Work out the finished part from the listing and answer in its coordinate system (mm). Face numbers are marked on the shaded views. A direction names the side the tool comes from. Coordinates: 2 decimals unless noted, no trailing zeros. Order: outer loops, then holes, each group sorted by start corner. A loop starts at its lowest first (then second) coordinate and runs counter-clockwise, first axis right, second up. Notation, with made-up numbers: (-37, 50) - (12, 50) arc R29 cw to (12, 81) - close; hole circle Ø4 at (76, -7.5). An arc over 180 degrees is marked (long way). Use CSV: the item, a comma, the result in double quotes. Start each with the question number.
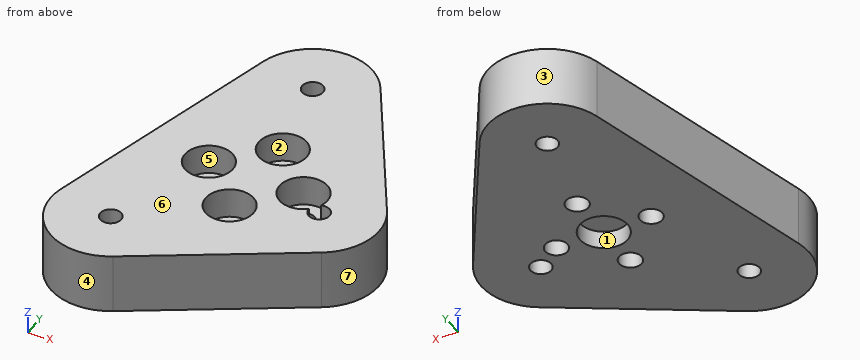
from build123d import *

# Parameters (mm, degrees)
SKETCH1_R               = 9
BOSS_EXTRUDE1_DEPTH     = 70
SKETCH2_R               = 2.5
CUT_EXTRUDE1_DEPTH      = 5
CUT_EXTRUDE2_REACH      = 90.987
CUT_EXTRUDE2_END_RADIUS = 9
SKETCH3_R               = 1.75
CIRPATTERN1_COUNT       = 3
SKETCH5_W               = 24.568161226
SKETCH5_H               = 25
SKETCH6_R               = 9
BOSS_EXTRUDE2_DEPTH     = 5
SKETCH8_R               = 9
SKETCH8_R_2             = 5.0505014
BOSS_EXTRUDE3_DEPTH     = 3
CUT_EXTRUDE3_REACH      = 83.112
SKETCH9_R               = 1.875
SKETCH11_R              = 4
CUT_EXTRUDE4_DEPTH      = 3
CUT_EXTRUDE5_DEPTH      = 82.111701173
CUT_EXTRUDE5_DEPTH_BACK = 82.111701173
SKETCH12_W              = 69.923732777
SKETCH12_H              = 71.865657343
SKETCH13_R              = 4
BOSS_EXTRUDE5_DEPTH     = 5
SKETCH14_R              = 1.75
CUT_EXTRUDE6_DEPTH      = 43.17947431


with BuildPart() as part:
    # Sketch1 → Boss-Extrude1 (new body)
    with BuildSketch(Plane.XY):
        with BuildLine():
            Line((-23.6546385, -16.539669722), (-13.23734813, 25.649078182))
            ThreePointArc((-13.23734813, 25.649078182), (-5.029445343, 33.138647287), (5.031042671, 28.421667909))
            Line((5.031042671, 28.421667909), (20.916771438, 2.118648772))
            ThreePointArc((20.916771438, 2.118648772), (22.065215706, -5.448366461), (17.526600651, -11.611126974))
            Line((17.526600651, -11.611126974), (-8.776418486, -27.496855741))
            ThreePointArc((-8.776418486, -27.496855741), (-19.876207308, -26.988917124), (-23.6546385, -16.539669722))
        make_face()
        Circle(SKETCH1_R, mode=Mode.SUBTRACT)
    extrude(amount=BOSS_EXTRUDE1_DEPTH)

    # Sketch2 → Cut-Extrude1 (cut)
    with BuildSketch(Plane(origin=(9.822624711, -16.263949206, 0), x_dir=(0.8559973266359324, 0.5169802479709809, 0), z_dir=(0.5169802479709809, -0.8559973266359324, 0))):
        with Locations((0, 65)):
            Circle(SKETCH2_R)
    cut_extrude1 = extrude(amount=-CUT_EXTRUDE1_DEPTH, mode=Mode.SUBTRACT)

    # Cut-Extrude2: up to this cylinder (the profile starts outside it)
    cut_extrude2_end = Plane(origin=(0, 0, 65), z_dir=(0, 0, -1)) * Cylinder(CUT_EXTRUDE2_END_RADIUS, 200.974, mode=Mode.PRIVATE)
    # Sketch3 → Cut-Extrude2 (cut, up to the surface)
    with BuildSketch(Plane(origin=(7.237723472, -11.983962573, 0), x_dir=(0.8559973266359324, 0.5169802479709809, 0), z_dir=(0.5169802479709809, -0.8559973266359324, 0)), mode=Mode.PRIVATE) as cut_extrude2_sk1:
        with Locations((0, 65)):
            Circle(SKETCH3_R)
    cut_extrude2_tool1 = extrude(cut_extrude2_sk1.sketch, amount=-CUT_EXTRUDE2_REACH, mode=Mode.PRIVATE) - cut_extrude2_end
    cut_extrude2 = cut_extrude2_tool1.solids().sort_by_distance((7.237723, -11.983963, 65))[0]
    add(cut_extrude2, mode=Mode.SUBTRACT)

    # CirPattern1: Cut-Extrude1, Cut-Extrude2 ×3 about axis
    cirpattern1_axis = Axis((0, 0, 0), (0, 0, 1))
    add([cut_extrude1.rotate(cirpattern1_axis, i * 360 / CIRPATTERN1_COUNT) for i in range(1, CIRPATTERN1_COUNT)], mode=Mode.SUBTRACT)
    add([cut_extrude2.rotate(cirpattern1_axis, i * 360 / CIRPATTERN1_COUNT) for i in range(1, CIRPATTERN1_COUNT)], mode=Mode.SUBTRACT)

    # Sketch5 → Cut-Revolve1 (revolve, cut)
    with BuildSketch(Plane(origin=(0, 0, 0), x_dir=(1, 0, 0), z_dir=(0, 1, 0)), mode=Mode.PRIVATE) as cut_revolve1_sk:
        with Locations((-12.284080613, -17.5)):
            Rectangle(SKETCH5_W, SKETCH5_H)
    revolve(cut_revolve1_sk.sketch.rotate(Axis((0, 0, 0), (0, 0, 1)), 180), axis=Axis((0, 0, 0), (0, 0, 1)), mode=Mode.SUBTRACT)

    # Sketch6 → Boss-Extrude2 (add)
    with BuildSketch(Plane(origin=(0, 0, 0), x_dir=(-1, 0, 0), z_dir=(0, 0, -1))):
        with Locations(Location((0, 0, 0), (0, 0, 180))):
            Circle(SKETCH6_R)
    extrude(amount=-BOSS_EXTRUDE2_DEPTH)

    # Sketch8 → Boss-Extrude3 (add)
    with BuildSketch(Plane(origin=(0, 0, 30), x_dir=(-1, 0, 0), z_dir=(0, 0, -1))):
        Circle(SKETCH8_R)
        Circle(SKETCH8_R_2, mode=Mode.SUBTRACT)
    extrude(amount=-BOSS_EXTRUDE3_DEPTH)

    # Sketch9 → Cut-Extrude3 (cut, up to next)
    with BuildSketch(Plane(origin=(0, 0, 0), x_dir=(-1, 0, 0), z_dir=(0, 0, -1)), mode=Mode.PRIVATE) as cut_extrude3_sk1:
        with Locations((0, 8)):
            Circle(SKETCH9_R)
    cut_extrude3_tool1 = extrude(cut_extrude3_sk1.sketch, amount=-CUT_EXTRUDE3_REACH, mode=Mode.PRIVATE) & part.part
    # Sketch9 → Cut-Extrude3 (cut, up to next)
    with BuildSketch(Plane(origin=(0, 0, 0), x_dir=(-1, 0, 0), z_dir=(0, 0, -1)), mode=Mode.PRIVATE) as cut_extrude3_sk2:
        with Locations((8, 0)):
            Circle(SKETCH9_R)
    cut_extrude3_tool2 = extrude(cut_extrude3_sk2.sketch, amount=-CUT_EXTRUDE3_REACH, mode=Mode.PRIVATE) & part.part
    # Sketch9 → Cut-Extrude3 (cut, up to next)
    with BuildSketch(Plane(origin=(0, 0, 0), x_dir=(-1, 0, 0), z_dir=(0, 0, -1)), mode=Mode.PRIVATE) as cut_extrude3_sk3:
        with Locations((0, -8)):
            Circle(SKETCH9_R)
    cut_extrude3_tool3 = extrude(cut_extrude3_sk3.sketch, amount=-CUT_EXTRUDE3_REACH, mode=Mode.PRIVATE) & part.part
    # Sketch9 → Cut-Extrude3 (cut, up to next)
    with BuildSketch(Plane(origin=(0, 0, 0), x_dir=(-1, 0, 0), z_dir=(0, 0, -1)), mode=Mode.PRIVATE) as cut_extrude3_sk4:
        with Locations((-8, 0)):
            Circle(SKETCH9_R)
    cut_extrude3_tool4 = extrude(cut_extrude3_sk4.sketch, amount=-CUT_EXTRUDE3_REACH, mode=Mode.PRIVATE) & part.part
    add(cut_extrude3_tool1.solids().sort_by_distance((0, 8, 0))[0], mode=Mode.SUBTRACT)
    add(cut_extrude3_tool2.solids().sort_by_distance((-8, 0, 0))[0], mode=Mode.SUBTRACT)
    add(cut_extrude3_tool3.solids().sort_by_distance((0, -8, 0))[0], mode=Mode.SUBTRACT)
    add(cut_extrude3_tool4.solids().sort_by_distance((8, 0, 0))[0], mode=Mode.SUBTRACT)

    # Sketch11 → Cut-Extrude4 (cut)
    with BuildSketch(Plane(origin=(0, 0, 0), x_dir=(-1, 0, 0), z_dir=(0, 0, -1))):
        Circle(SKETCH11_R)
    extrude(amount=-CUT_EXTRUDE4_DEPTH, mode=Mode.SUBTRACT)

    # Sketch12 → Cut-Extrude5 (cut, two sides: drawn at the far end of the back side and taken through both)
    with BuildSketch(Plane(origin=(0, 0, 0), x_dir=(0, 0, -1), z_dir=(1, 0, 0)).offset(-CUT_EXTRUDE5_DEPTH_BACK)):
        with Locations((-39.961866388, -0.358209869)):
            Rectangle(SKETCH12_W, SKETCH12_H)
    extrude(amount=CUT_EXTRUDE5_DEPTH + CUT_EXTRUDE5_DEPTH_BACK, mode=Mode.SUBTRACT)

    # Sketch13 → Boss-Extrude5 (add)
    with BuildSketch(Plane.XY.offset(5)):
        with BuildLine():
            Line((-8.776418486, -27.496855741), (17.526600651, -11.611126974))
            ThreePointArc((17.526600651, -11.611126974), (22.065215706, -5.448366461), (20.916771438, 2.118648772))
            Line((20.916771438, 2.118648772), (5.031042671, 28.421667909))
            ThreePointArc((5.031042671, 28.421667909), (-5.029445343, 33.138647287), (-13.23734813, 25.649078182))
            Line((-13.23734813, 25.649078182), (-23.6546385, -16.539669722))
            ThreePointArc((-23.6546385, -16.539669722), (-19.876207308, -26.988917124), (-8.776418486, -27.496855741))
        make_face()
        with Locations((-8, 0)):
            Circle(SKETCH13_R, mode=Mode.SUBTRACT)
        with Locations((0, 8)):
            Circle(SKETCH13_R, mode=Mode.SUBTRACT)
        with Locations((8, 0)):
            Circle(SKETCH13_R, mode=Mode.SUBTRACT)
        with Locations((0, -8)):
            Circle(SKETCH13_R, mode=Mode.SUBTRACT)
    extrude(amount=BOSS_EXTRUDE5_DEPTH)

    # Sketch14 → Cut-Extrude6 (cut, through all)
    with BuildSketch(Plane(origin=(0, 0, 0), x_dir=(-1, 0, 0), z_dir=(0, 0, -1))):
        with Locations((3.528930595, 23.25186543)):
            Circle(SKETCH14_R)
        with Locations((-12.356798171, -3.051153708)):
            Circle(SKETCH14_R)
        with Locations((13.946220966, -18.936882475)):
            Circle(SKETCH14_R)
    extrude(amount=-CUT_EXTRUDE6_DEPTH, mode=Mode.SUBTRACT)


solid = part.part
1) The part is cut by section D-D on y = 0. Determine the outline of the cut face in (x, z) (3 decimals).
2) The part is cut by section C-C on x = -8. Determine the outline of the cut face in (y, z) (3 decimals).
3) The part is cut by section A-A on x = 0. Determine the outline of the cut face in (y, z) (1 decimal), plus the area to 3 significant figures.
4) For the marked faces 1, 2 and 3, determine the directions among +Z, -Z, +X, -X, +Y, -Y from which every point of the face is accessible in a straight line to the end or side of a thin tool.
5) Straight lines are drawn through the part: line 1 (Y direction, x = 0, z = 3.7) (1 decimal); line 2 (Y direction, x = 6, z = 8.25); line 3 (Z direction, x = 3, y = 6.5). For each, find the intervals that lie inside material, in ascending order. Write a range as [from, to].
6) For a pull along X with two mould halves and no side action, classify the marked faces 4, 5, 6 and 7 as +X half, -X half, draft (parallel to the pull), parting line (faces both ways), or undercut.
7) The part is cut by section B-B on y = 8. Determine the outline of the cut face in (x, z) (3 decimals), plus the area to 3 significant figures.
8) Flat-ended cylindrical pins translate along their axes: P1, Ø4.5, axis at x = 8, y = 0, coming from the +Z side; P2, Ø3, axis at x = -3.53, y = 23.25, coming from the -Z side; P3, Ø1.5, axis at y = 2.5, z = 2, coming from the -X side; P4, Ø4, axis at y = 20.5, z = 3, coming from the -X side. Find the tip coordinate at first contact, or state that the pin passes through.
Answer key:
1,outline,"(-19.571, 0) - (-9.875, 0) - (-9.875, 5) - (-12, 5) - (-12, 10) - (-19.571, 10) - close; (-6.125, 0) - (-4, 0) - (-4, 3) - (4, 3) - (4, 0) - (6.125, 0) - (6.125, 5) - (4, 5) - (4, 10) - (-4, 10) - (-4, 5) - (-6.125, 5) - close; (9.875, 0) - (21.88, 0) - (21.88, 10) - (12, 10) - (12, 5) - (9.875, 5) - close"
2,outline,"(-27.028, 0) - (-1.875, 0) - (-1.875, 5) - (-4, 5) - (-4, 10) - (-27.028, 10) - close; (1.875, 0) - (32.197, 0) - (32.197, 10) - (4, 10) - (4, 5) - (1.875, 5) - close"
3,outline,"(-22.2, 0) - (-9.9, 0) - (-9.9, 5) - (-12, 5) - (-12, 10) - (-22.2, 10) - close; (-6.1, 0) - (-4, 0) - (-4, 3) - (4, 3) - (4, 0) - (6.1, 0) - (6.1, 5) - (4, 5) - (4, 10) - (-4, 10) - (-4, 5) - (-6.1, 5) - close; (9.9, 0) - (32.6, 0) - (32.6, 10) - (12, 10) - (12, 5) - (9.9, 5) - close"
3,area,"407 mm^2"
4,face 1,"-Z"
4,face 2,"+Z"
4,face 3,"+Z, -Z, +Y"
5,line 1,"[-22.2, -9.9], [-6.1, 6.1], [9.9, 32.6]"
5,line 2,"[-18.57, -3.46], [3.46, 26.82]"
5,line 3,"[0, 5]"
6,face 4,"parting line"
6,face 5,"undercut"
6,face 6,"draft"
6,face 7,"+X half"
7,outline,"(-17.595, 0) - (-1.875, 0) - (-1.875, 5) - (-4, 5) - (-4, 10) - (-17.595, 10) - close; (1.875, 0) - (17.365, 0) - (17.365, 10) - (4, 10) - (4, 5) - (1.875, 5) - close"
7,area,"291 mm^2"
8,P1,"z = 5"
8,P2,"through"
8,P3,"x = -19.14"
8,P4,"x = -15"
